Design review of the part built by this model. Coordinates are the model's own, in mm. A direction names the side the tool comes from. Coordinates: 2 decimals unless noted, no trailing zeros. Loops run counter-clockwise (first coordinate to the right, second up) from the corner with the lowest first, then second, coordinate; pieces in that order, holes last. Notation, with made-up numbers: M 60,-38 L 119,-38 A27 ccw 119,1 Z; hole C 20.25,25 d8. An arc over 180 degrees is marked long. Write item = value, one per line. Start each with the question number.
from build123d import *

# Parameters (mm, degrees)
SKETCH1_W                      = 125
SKETCH1_H                      = 95
SKETCH1_R                      = 8.5
BOSS_EXTRUDE1_DEPTH            = 30
M4X0_7_TAPPED_HOLE1_AT_2_COUNT = 2
M4X0_7_TAPPED_HOLE1_AT_2_PITCH = 26.870057685
M4X0_7_TAPPED_HOLE1_AT_3_COUNT = 2
M4X0_7_TAPPED_HOLE1_AT_3_PITCH = 38
M4X0_7_TAPPED_HOLE1_AT_4_COUNT = 2
M4X0_7_TAPPED_HOLE1_AT_4_PITCH = 26.870057685
LPATTERN1_COUNT                = 2
LPATTERN1_PITCH                = 88
LPATTERN1_COUNT_DIR2           = 2
LPATTERN1_PITCH_DIR2           = 58
SKETCH5_W                      = 60
SKETCH5_H                      = 60
CUT_EXTRUDE1_DEPTH             = 20
FILLET1_R                      = 7
FILLET2_R                      = 3
F_1_4_20_TAPPED_HOLE1_D        = 5.1054
SKETCH8_R                      = 5
CUT_EXTRUDE2_DEPTH             = 31
M4_CLEARANCE_HOLE1_D           = 4.5


with BuildPart() as part:
    # Sketch1 → Boss-Extrude1 (new body)
    with BuildSketch(Plane(origin=(0, 0, 0), x_dir=(1, 0, 0), z_dir=(0, 1, 0))):
        Rectangle(SKETCH1_W, SKETCH1_H)
        with Locations((-44, 29)):
            Circle(SKETCH1_R, mode=Mode.SUBTRACT)
        with Locations((44, 29)):
            Circle(SKETCH1_R, mode=Mode.SUBTRACT)
        with Locations((44, -29)):
            Circle(SKETCH1_R, mode=Mode.SUBTRACT)
        with Locations((-44, -29)):
            Circle(SKETCH1_R, mode=Mode.SUBTRACT)
    extrude(amount=BOSS_EXTRUDE1_DEPTH)

    # Sketch2 → M4x0.7 Tapped Hole1 (revolve, cut)
    with BuildSketch(Plane(origin=(-57.435028843, 30, -42.435028843), x_dir=(0, 0, 1), z_dir=(1, 0, 0))):
        Polygon((0, 0), (0, 8.991420021), (1.65, 8), (1.65, 0), align=None)
    m4x0_7_tapped_hole1 = revolve(axis=Axis((-57.435028843, 36.35, -42.435028843), (0, -1, 0)), mode=Mode.SUBTRACT)

    # M4x0.7 Tapped Hole1 at 2: M4x0.7 Tapped Hole1 ×2
    with Locations(*[(i * M4X0_7_TAPPED_HOLE1_AT_2_PITCH, 0, 0) for i in range(1, M4X0_7_TAPPED_HOLE1_AT_2_COUNT)]):
        add(m4x0_7_tapped_hole1, mode=Mode.SUBTRACT)

    # M4x0.7 Tapped Hole1 at 3: M4x0.7 Tapped Hole1 ×2
    with Locations(*[Vector(0.707106781, 0, 0.707106781) * (i * M4X0_7_TAPPED_HOLE1_AT_3_PITCH) for i in range(1, M4X0_7_TAPPED_HOLE1_AT_3_COUNT)]):
        add(m4x0_7_tapped_hole1, mode=Mode.SUBTRACT)

    # M4x0.7 Tapped Hole1 at 4: M4x0.7 Tapped Hole1 ×2
    with Locations(*[(0, 0, i * M4X0_7_TAPPED_HOLE1_AT_4_PITCH) for i in range(1, M4X0_7_TAPPED_HOLE1_AT_4_COUNT)]):
        add(m4x0_7_tapped_hole1, mode=Mode.SUBTRACT)

    # LPattern1: M4x0.7 Tapped Hole1 2 × 2
    with Locations(*[(i * LPATTERN1_PITCH, 0, j * LPATTERN1_PITCH_DIR2) for i in range(LPATTERN1_COUNT) for j in range(LPATTERN1_COUNT_DIR2) if (i, j) != (0, 0)]):
        add(m4x0_7_tapped_hole1, mode=Mode.SUBTRACT)

    # LPattern1 copy 1 sketch → LPattern1 copy 1 (revolve, cut)
    with BuildSketch(Plane(origin=(-30.564971157, 30, 15.564971157), x_dir=(0, 0, 1), z_dir=(1, 0, 0))):
        Polygon((0, 0), (0, 8.991420021), (1.65, 8), (1.65, 0), align=None)
    revolve(axis=Axis((-30.564971157, 36.35, 15.564971157), (0, -1, 0)), mode=Mode.SUBTRACT)

    # LPattern1 copy 2 sketch → LPattern1 copy 2 (revolve, cut)
    with BuildSketch(Plane(origin=(57.435028843, 30, -42.435028843), x_dir=(0, 0, 1), z_dir=(1, 0, 0))):
        Polygon((0, 0), (0, 8.991420021), (1.65, 8), (1.65, 0), align=None)
    revolve(axis=Axis((57.435028843, 36.35, -42.435028843), (0, -1, 0)), mode=Mode.SUBTRACT)

    # LPattern1 copy 3 sketch → LPattern1 copy 3 (revolve, cut)
    with BuildSketch(Plane(origin=(57.435028843, 30, 15.564971157), x_dir=(0, 0, 1), z_dir=(1, 0, 0))):
        Polygon((0, 0), (0, 8.991420021), (1.65, 8), (1.65, 0), align=None)
    revolve(axis=Axis((57.435028843, 36.35, 15.564971157), (0, -1, 0)), mode=Mode.SUBTRACT)

    # LPattern1 copy 4 sketch → LPattern1 copy 4 (revolve, cut)
    with BuildSketch(Plane(origin=(-30.564971157, 30, 42.435028843), x_dir=(0, 0, 1), z_dir=(1, 0, 0))):
        Polygon((0, 0), (0, 8.991420021), (1.65, 8), (1.65, 0), align=None)
    revolve(axis=Axis((-30.564971157, 36.35, 42.435028843), (0, -1, 0)), mode=Mode.SUBTRACT)

    # LPattern1 copy 5 sketch → LPattern1 copy 5 (revolve, cut)
    with BuildSketch(Plane(origin=(57.435028843, 30, -15.564971157), x_dir=(0, 0, 1), z_dir=(1, 0, 0))):
        Polygon((0, 0), (0, 8.991420021), (1.65, 8), (1.65, 0), align=None)
    revolve(axis=Axis((57.435028843, 36.35, -15.564971157), (0, -1, 0)), mode=Mode.SUBTRACT)

    # LPattern1 copy 6 sketch → LPattern1 copy 6 (revolve, cut)
    with BuildSketch(Plane(origin=(57.435028843, 30, 42.435028843), x_dir=(0, 0, 1), z_dir=(1, 0, 0))):
        Polygon((0, 0), (0, 8.991420021), (1.65, 8), (1.65, 0), align=None)
    revolve(axis=Axis((57.435028843, 36.35, 42.435028843), (0, -1, 0)), mode=Mode.SUBTRACT)

    # LPattern1 copy 7 sketch → LPattern1 copy 7 (revolve, cut)
    with BuildSketch(Plane(origin=(-57.435028843, 30, 42.435028843), x_dir=(0, 0, 1), z_dir=(1, 0, 0))):
        Polygon((0, 0), (0, 8.991420021), (1.65, 8), (1.65, 0), align=None)
    revolve(axis=Axis((-57.435028843, 36.35, 42.435028843), (0, -1, 0)), mode=Mode.SUBTRACT)

    # LPattern1 copy 8 sketch → LPattern1 copy 8 (revolve, cut)
    with BuildSketch(Plane(origin=(30.564971157, 30, -15.564971157), x_dir=(0, 0, 1), z_dir=(1, 0, 0))):
        Polygon((0, 0), (0, 8.991420021), (1.65, 8), (1.65, 0), align=None)
    revolve(axis=Axis((30.564971157, 36.35, -15.564971157), (0, -1, 0)), mode=Mode.SUBTRACT)

    # LPattern1 copy 9 sketch → LPattern1 copy 9 (revolve, cut)
    with BuildSketch(Plane(origin=(30.564971157, 30, 42.435028843), x_dir=(0, 0, 1), z_dir=(1, 0, 0))):
        Polygon((0, 0), (0, 8.991420021), (1.65, 8), (1.65, 0), align=None)
    revolve(axis=Axis((30.564971157, 36.35, 42.435028843), (0, -1, 0)), mode=Mode.SUBTRACT)

    # Sketch5 → Cut-Extrude1 (cut)
    with BuildSketch(Plane.XZ):
        Rectangle(SKETCH5_W, SKETCH5_H)
    extrude(amount=-CUT_EXTRUDE1_DEPTH, mode=Mode.SUBTRACT)

    # Fillet1
    fillet1_edges = [part.edges().sort_by_distance(p)[0] for p in [
        (-30, 10, -30),
        (-30, 10, 30),
        (30, 10, 30),
        (30, 10, -30),
    ]]
    fillet(fillet1_edges, radius=FILLET1_R)

    # Fillet2
    fillet2_edges = [part.edges().sort_by_distance(p)[0] for p in [
        (-62.5, 15, -47.5),
        (62.5, 15, -47.5),
        (62.5, 15, 47.5),
        (-62.5, 15, 47.5),
    ]]
    fillet(fillet2_edges, radius=FILLET2_R)

    # 1/4-20 Tapped Hole1 (through all)
    with Locations(Plane(origin=(0, 20, 0), x_dir=(-1, 0, 0), z_dir=(0, -1, 0))):
        with Locations((0, 0)):
            Hole(F_1_4_20_TAPPED_HOLE1_D / 2)

    # Sketch8 → Cut-Extrude2 (cut, through all)
    with BuildSketch(Plane.XZ):
        with Locations((-15, 15)):
            Circle(SKETCH8_R)
        with Locations((-15, -15)):
            Circle(SKETCH8_R)
        with Locations((15, 15)):
            Circle(SKETCH8_R)
        with Locations((15, -15)):
            Circle(SKETCH8_R)
    extrude(amount=-CUT_EXTRUDE2_DEPTH, mode=Mode.SUBTRACT)

    # M4 Clearance Hole1 (through all)
    with Locations(Plane(origin=(0, 20, 0), x_dir=(-1, 0, 0), z_dir=(0, -1, 0))):
        with Locations((22, -22), (-22, -22), (-22, 22), (22, 22)):
            Hole(M4_CLEARANCE_HOLE1_D / 2)


solid = part.part
Q1. Add section B-B on z = 33. State the section outline as (x, y) points, plus the area to 3 significant figures.
Q2. For faces 1 (the face through (0, 10, 30)), 2 (the face through (61.6, 15.21, -46.64)), 3 (the face through (-55.824, 26.056, -42.793)), list the 3-axis set-ups (+Z, -Z, +X, -X, +Y, -Y) from which the entire face can be reached by the end or side of a thin tool; tool diameter is ignored.
Q3. Clearance check with flat-ended pins moving along their axes: P1, Ø2, axis at x = -57.44, z = 42.44, coming from the +Y side; P2, Ø13.5, axis at x = -44, z = -29, coming from the +Y side; P3, Ø5, axis at x = 21.5, z = -10, coming from the -Y side. State where each tip first meets the part, or that it passes through.
Q4. Add section A-A on x = 0. State the section outline as (y, z) points.
Q5. Add section C-C on y = 7.75. State the section outline as (x, z) points, plus the area to 3 significant figures.
Q6. Add section D-D on x = 44. State the section outline as (y, z) points.
Q7. Mouldability with a two-part tool opening along X and no side actions: class faces 4 (the face through (-20.962, 25.07, -20.004)), 5 (the face through (-61.64, 15.21, -46.6)), 6 (the face through (-1, 0, 31)) as released by +X, released by -X, zero draft, split by the parting line, or undercut.
Q8. To check wall thickness, follow line 1 (Z direction, x = 44, y = 10.5); line 2 (Z direction, x = -22, y = 26); line 3 (Z direction, x = 10.5, y = 9.75). State the ranges of each line that lie inside material, in increasing order. Write a range as from..to.
Values follow:
q1.outline = M -62.5,0 L -51.5,0 L -51.5,30 L -62.5,30 Z; M -36.5,0 L 36.5,0 L 36.5,30 L -36.5,30 Z; M 51.5,0 L 62.5,0 L 62.5,30 L 51.5,30 Z
q1.area = 2,850 mm2
q2.face_1 = -Y
q2.face_2 = -Z, +X, +Y, -Y
q2.face_3 = +Y
q3.P1 = 21.61
q3.P2 = through
q3.P3 = 20
q4.outline = M 0,-47.5 L 30,-47.5 L 30,-2.55 L 20,-2.55 L 20,-30 L 0,-30 Z; M 0,30 L 20,30 L 20,2.55 L 30,2.55 L 30,47.5 L 0,47.5 Z
q5.outline = M -62.5,-44.5 A3 ccw -59.5,-47.5 L 59.5,-47.5 A3 ccw 62.5,-44.5 L 62.5,44.5 A3 ccw 59.5,47.5 L -59.5,47.5 A3 ccw -62.5,44.5 Z; hole C -44,-29 d17; hole C -44,29 d17; hole M -30,-23 A7 ccw -23,-30 L 23,-30 A7 ccw 30,-23 L 30,23 A7 ccw 23,30 L -23,30 A7 ccw -30,23 Z; hole C 44,-29 d17; hole C 44,29 d17
q5.area = 7,400 mm2
q6.outline = M 0,-47.5 L 30,-47.5 L 30,-37.5 L 0,-37.5 Z; M 0,-20.5 L 30,-20.5 L 30,20.5 L 0,20.5 Z; M 0,37.5 L 30,37.5 L 30,47.5 L 0,47.5 Z
q7.face_4 = undercut
q7.face_5 = released by -X
q7.face_6 = zero draft
q8.line_1 = -47.5..-37.5, -20.5..20.5, 37.5..47.5
q8.line_2 = -47.5..-24.25, -19.75..19.75, 24.25..47.5
q8.line_3 = -47.5..-30, 30..47.5
